from build123d import *

# Parameters (mm, degrees)
SKETCH1_W               = 100
SKETCH1_H               = 90
BOSS_EXTRUDE1_DEPTH     = 5
FILLET1_R               = 5
FILLET2_R               = 5
SKETCH2_R               = 1.55
CUT_EXTRUDE1_DEPTH      = 10
SKETCH3_R               = 3
CUT_EXTRUDE2_DEPTH      = 2.5
SKETCH4_R               = 1.5
SKETCH4_W               = 71
SKETCH4_H               = 26
CUT_EXTRUDE3_DEPTH      = 135.629120178
SKETCH5_R               = 1.5
CUT_EXTRUDE4_DEPTH      = 135.629120178
SKETCH8_R               = 3.75
BOSS_EXTRUDE3_DEPTH     = 7.5
SKETCH6_R               = 3
CUT_EXTRUDE5_DEPTH      = 2.5
CUT_EXTRUDE7_DEPTH      = 135.745129782
CUT_EXTRUDE7_DEPTH_BACK = 135.745129782
SKETCH10_R              = 1.55
SKETCH11_R              = 6
SKETCH11_R_2            = 3
CUT_EXTRUDE8_DEPTH      = 5


with BuildPart() as part:
    # Sketch1 → Boss-Extrude1 (new body)
    with BuildSketch(Plane(origin=(0, 0, 0), x_dir=(1, 0, 0), z_dir=(0, 1, 0))):
        with Locations((50, 45)):
            Rectangle(SKETCH1_W, SKETCH1_H)
    extrude(amount=BOSS_EXTRUDE1_DEPTH)

    # Fillet1
    fillet1_edges = [part.edges().sort_by_distance(p)[0] for p in [
        (0, 2.5, -90),
        (100, 2.5, -90),
        (100, 2.5, 0),
        (0, 2.5, 0),
    ]]
    fillet(fillet1_edges, radius=FILLET1_R)

    # Fillet2
    fillet2_edges = [part.edges().sort_by_distance(p)[0] for p in [
        (1.464466094, 5, -1.464466094),
        (98.535533906, 5, -88.535533906),
        (98.535533906, 5, -1.464466094),
        (100, 5, -45),
        (50, 5, 0),
        (0, 5, -45),
        (1.464466094, 5, -88.535533906),
        (50, 5, -90),
    ]]
    fillet(fillet2_edges, radius=FILLET2_R - 0.0001)  # a hair under: the kernel refuses the full size

    # Sketch2 → Cut-Extrude1 (cut)
    with BuildSketch(Plane(origin=(0, 5, 0), x_dir=(1, 0, 0), z_dir=(0, 1, 0))):
        with Locations(Location((10, 80, 0), (0, 0, 270))):
            Circle(SKETCH2_R)
        with Locations(Location((10, 10, 0), (0, 0, 270))):
            Circle(SKETCH2_R)
        with Locations(Location((90, 10, 0), (0, 0, 270))):
            Circle(SKETCH2_R)
        with Locations(Location((90, 80, 0), (0, 0, 270))):
            Circle(SKETCH2_R)
    extrude(amount=-CUT_EXTRUDE1_DEPTH, mode=Mode.SUBTRACT)

    # Sketch3 → Cut-Extrude2 (cut)
    with BuildSketch(Plane(origin=(0, 5, 0), x_dir=(1, 0, 0), z_dir=(0, 1, 0))):
        with Locations(Location((10, 80, 0), (0, 0, 270))):
            Circle(SKETCH3_R)
        with Locations(Location((90, 80, 0), (0, 0, 270))):
            Circle(SKETCH3_R)
        with Locations(Location((90, 10, 0), (0, 0, 270))):
            Circle(SKETCH3_R)
        with Locations(Location((10, 10, 0), (0, 0, 270))):
            Circle(SKETCH3_R)
    extrude(amount=-CUT_EXTRUDE2_DEPTH, mode=Mode.SUBTRACT)

    # Sketch4 → Cut-Extrude3 (cut, through all)
    with BuildSketch(Plane(origin=(0, 5, 0), x_dir=(1, 0, 0), z_dir=(0, 1, 0))):
        with Locations(Location((35, 29, 0), (0, 0, 270))):
            Circle(SKETCH4_R)
        with Locations(Location((40, 29, 0), (0, 0, 270))):
            Circle(SKETCH4_R)
        with Locations(Location((50, 29, 0), (0, 0, 270))):
            Circle(SKETCH4_R)
        with Locations(Location((55, 29, 0), (0, 0, 270))):
            Circle(SKETCH4_R)
        with Locations(Location((65, 29, 0), (0, 0, 270))):
            Circle(SKETCH4_R)
        with Locations((50, 52)):
            Rectangle(SKETCH4_W, SKETCH4_H)
    extrude(amount=-CUT_EXTRUDE3_DEPTH, mode=Mode.SUBTRACT)

    # Sketch5 → Cut-Extrude4 (cut, through all)
    with BuildSketch(Plane.XZ):
        with Locations(Location((9, -39.5, 0), (0, 0, 270))):
            Circle(SKETCH5_R)
        with Locations(Location((9, -64.5, 0), (0, 0, 270))):
            Circle(SKETCH5_R)
        with Locations(Location((91, -64.5, 0), (0, 0, 270))):
            Circle(SKETCH5_R)
        with Locations(Location((91, -39.5, 0), (0, 0, 270))):
            Circle(SKETCH5_R)
    extrude(amount=-CUT_EXTRUDE4_DEPTH, mode=Mode.SUBTRACT)

    # Sketch8 → Boss-Extrude3 (add)
    with BuildSketch(Plane.XZ):
        with Locations(Location((8.75, -39.5, 0), (0, 0, 270))):
            Circle(SKETCH8_R)
        with Locations(Location((91.25, -39.5, 0), (0, 0, 270))):
            Circle(SKETCH8_R)
        with Locations(Location((91.25, -64.5, 0), (0, 0, 270))):
            Circle(SKETCH8_R)
        with Locations(Location((8.75, -64.5, 0), (0, 0, 270))):
            Circle(SKETCH8_R)
    extrude(amount=BOSS_EXTRUDE3_DEPTH)

    # Sketch6 → Cut-Extrude5 (cut)
    with BuildSketch(Plane(origin=(0, 5, 0), x_dir=(1, 0, 0), z_dir=(0, 1, 0))):
        with Locations(Location((9, 39.5, 0), (0, 0, 270))):
            Circle(SKETCH6_R)
        with Locations(Location((9, 64.5, 0), (0, 0, 270))):
            Circle(SKETCH6_R)
        with Locations(Location((91, 64.5, 0), (0, 0, 270))):
            Circle(SKETCH6_R)
        with Locations(Location((91, 39.5, 0), (0, 0, 270))):
            Circle(SKETCH6_R)
    extrude(amount=-CUT_EXTRUDE5_DEPTH, mode=Mode.SUBTRACT)

    # Sketch10 → Cut-Extrude7 (cut, two sides: drawn at the far end of the back side and taken through both)
    with BuildSketch(Plane(origin=(0, 0, 0), x_dir=(1, 0, 0), z_dir=(0, 1, 0)).offset(-CUT_EXTRUDE7_DEPTH_BACK)):
        with Locations(Location((9, 64.5, 0), (0, 0, 270))):
            Circle(SKETCH10_R)
        with Locations(Location((9, 39.5, 0), (0, 0, 270))):
            Circle(SKETCH10_R)
        with Locations(Location((91, 39.5, 0), (0, 0, 270))):
            Circle(SKETCH10_R)
        with Locations(Location((91, 64.5, 0), (0, 0, 270))):
            Circle(SKETCH10_R)
    extrude(amount=CUT_EXTRUDE7_DEPTH + CUT_EXTRUDE7_DEPTH_BACK, mode=Mode.SUBTRACT)

    # Sketch11 → Cut-Extrude8 (cut)
    with BuildSketch(Plane(origin=(0, 5, 0), x_dir=(1, 0, 0), z_dir=(0, 1, 0))):
        with Locations(Location((37.5, 16.5, 0), (0, 0, 270))):
            Circle(SKETCH11_R)
        with Locations(Location((65, 16.5, 0), (0, 0, 270))):
            Circle(SKETCH11_R_2)
    extrude(amount=-CUT_EXTRUDE8_DEPTH, mode=Mode.SUBTRACT)


solid = part.part
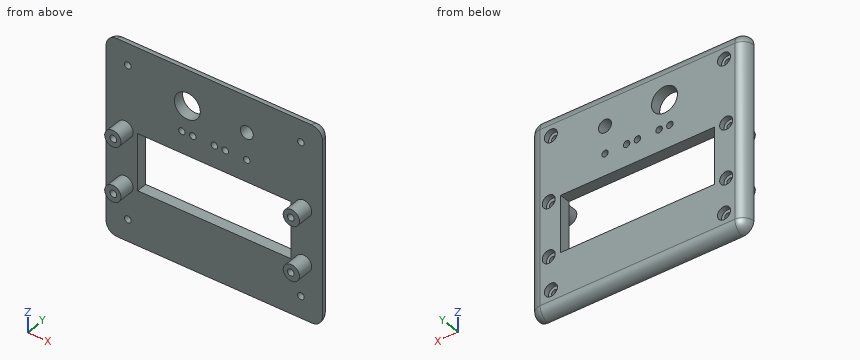
Can you work these out from the model? Positions are in its coordinate system, mm. Round coordinates to 2 decimals unless told otherwise and drop trailing zeros. Order: outer loops, then holes, each group sorted by start corner. A loop starts at its lowest first (then second) coordinate and runs counter-clockwise, first axis right, second up. Notation, with made-up numbers: (75.5, -5) -> (134.5, -5) arc R20 ccw to (134.5, 19) -> close; hole circle Ø2 at (81, 4). An arc over 180 degrees is marked (long way). Write each question's results on one line, items separated by ' | '. Start each with the question number.
Item 1: If we section it at A-A, the plane y = -2: Write out the boundary of the cut face in (x, z).
Item 2: If we section it at B-B, the plane x = 50: State how many separate pieces and enclosed holes the cut face has, then the cut area to 3 significant figures.
Item 3: Please list where these lines run through material, in increasing order: L1, parallel to X at y = -0.5, z = -39.5; L2, parallel to X at y = 2.3, z = -29; L3, parallel to X at y = 0.25, z = -53.5.
Item 4: Will these pins go through, and if not, where does the flat tip stop? pin 1 (4 mm diameter, centred on x = 90, z = -10, fed in from +Y); pin 2 (5.5 mm diameter, centred on y = 3.5, z = -45.5, fed in from +X); pin 3 (3 mm diameter, centred on x = 51, y = 2.5, fed in from +Z).
Results:
1) outline: circle Ø7.5 at (8.75, -64.5); circle Ø7.5 at (8.75, -39.5); circle Ø7.5 at (91.25, -64.5); circle Ø7.5 at (91.25, -39.5); hole circle Ø3.1 at (9, -64.5); hole circle Ø3.1 at (9, -39.5); hole circle Ø3.1 at (91, -64.5); hole circle Ø3.1 at (91, -39.5)
2) separate pieces: 3 | enclosed holes: 0 | area: 294 mm2
3) L1: x = 5 to 7.45, 10.55 to 12.5, 87.5 to 89.45, 92.55 to 95 | L2: x = 0.56 to 33.5, 36.5 to 38.5, 41.5 to 48.5, 51.5 to 53.5, 56.5 to 63.5, 66.5 to 99.44 | L3: x = 0.01 to 14.5, 85.5 to 99.99
4) pin 1: stops at y = 2.5 | pin 2: stops at x = 99.94 | pin 3: stops at z = -0.1
